Work out the finished part from the listing and answer in its coordinate system (mm). Face numbers are marked on the shaded views. A direction names the side the tool comes from. Coordinates: 2 decimals unless noted, no trailing zeros. Order: outer loops, then holes, each group sorted by start corner. A loop starts at its lowest first (then second) coordinate and runs counter-clockwise, first axis right, second up. Notation, with made-up numbers: (49, 60.5) -> (66, 60.5) arc R24 cw to (66, 91.5) -> close; hole circle Ø4 at (55, 6). An arc over 180 degrees is marked (long way). Answer as CSV lines item,"result". Start each with the question number.
Item 1: Section B-B (y = -30) is taken. Write down the section's boundary in (x, z), then the cut area to 3 significant figures.
Item 2: Which of the six approach directions +Z, -Z, +X, -X, +Y, -Y give full straight-line access (tool end or side, diameter ignored) to the marked faces 1 and 2?
Item 3: Section D-D (y = -9) is taken. Write down the section's boundary in (x, z).
Item 4: For a pull along Z with two mould halves and no side action, classify the marked faces 3, 4, 5 and 6 as pulls with the +Z half, pulls with the -Z half, needs draft (parallel to the pull), parting line crosses it, or undercut.
Item 5: Straight lines are drawn through the part: L1, parallel to X at y = -28, z = 0; L2, parallel to Z at x = -22.5, y = -33; L3, parallel to X at y = -10, z = 19. For each, find the intervals that lie inside material, in ascending order.
Item 6: Section C-C (x = -26) is taken. Write down the section's boundary in (y, z).
Item 7: Each of these flat-tipped pins is pushed along its axis until it touches: pin 1 Ø12 at (x, z) = (-53.5, -6.5) entering from -Y; pin 2 Ø12 at (y, z) = (-39, 24) entering from -X; pin 3 Ø8 at (y, z) = (-53, 54) entering from -X. Where does it stop, or does it pass through?
Item 8: Section A-A (z = 0) is taken. Write down the section's boundary in (x, y), then the cut area to 3 significant figures.
```python
from build123d import *

# Parameters (mm, degrees)
F0_W     = 10
F0_H     = 30
F1_DEPTH = 60
F2_R     = 10.2
F3_DEPTH = 80
F4_SIZE2 = 5
F4_SIZE  = 1


with BuildPart() as f1:
    # F0 (on Front) → F1 (new body)
    with BuildSketch(Plane.XZ):
        Polygon((5.41889066, 74.0884651807), (-5, 15), (5, 15), (15.41889066, 74.0884651807), align=None)
        Rectangle(F0_W, F0_H)
        Polygon((5, -15), (-5, -15), (5.41889066, -74.0884651807), (15.41889066, -74.0884651807), align=None)
    extrude(amount=F1_DEPTH)

    # F2 (on face) → F3 (join)
    with BuildSketch(Plane(origin=(-5, 0, 0), x_dir=(0, -1, 0), z_dir=(-1, 0, 0))):
        with Locations((30, 0)):
            Circle(F2_R)
    extrude(amount=F3_DEPTH)

    # F4
    f4_edges = [f1.edges().sort_by_distance(p)[0] for p in [
        (-85, -19.8, 0),
    ]]
    f4_side = f1.faces().sort_by_distance((-85, -30, 0))[0]
    chamfer(f4_edges, length=F4_SIZE, length2=F4_SIZE2, reference=f4_side)


solid = f1.part
```
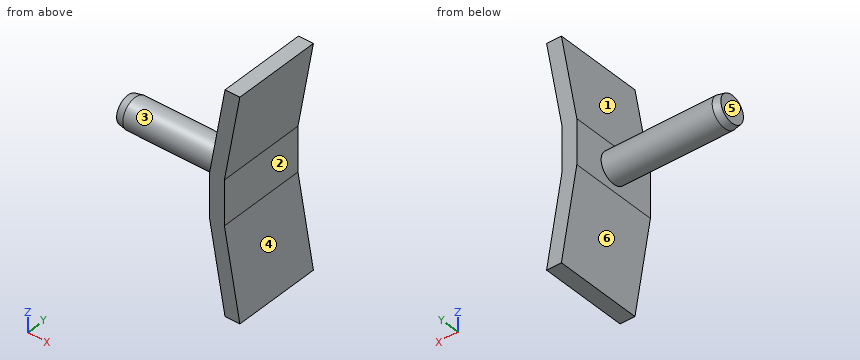
Checked values:
1,outline,"(-85, -9.2) -> (-80, -10.2) -> (-5, -10.2) -> (-5, -15) -> (5.42, -74.09) -> (15.42, -74.09) -> (5, -15) -> (5, 15) -> (15.42, 74.09) -> (5.42, 74.09) -> (-5, 15) -> (-5, 10.2) -> (-80, 10.2) -> (-85, 9.2) -> close"
1,area,"3,110 mm^2"
2,face 1,"+Z, -X, +Y, -Y"
2,face 2,"+X, +Y, -Y"
3,outline,"(-5, -15) -> (5.42, -74.09) -> (15.42, -74.09) -> (5, -15) -> (5, 15) -> (15.42, 74.09) -> (5.42, 74.09) -> (-5, 15) -> close"
4,face 3,"parting line crosses it"
4,face 4,"undercut"
4,face 5,"needs draft"
4,face 6,"pulls with the -Z half"
5,L1,"x = -85 to 5"
5,L2,"z = -9.75 to 9.75"
5,L3,"x = -4.29 to 5.71"
6,outline,"circle Ø20.4 at (-30, 0)"
7,pin 1,"stops at y = -40.19"
7,pin 2,"stops at x = -4.47"
7,pin 3,"stops at x = 1.17"
8,outline,"(-85, -39.2) -> (-80, -40.2) -> (-5, -40.2) -> (-5, -60) -> (5, -60) -> (5, 0) -> (-5, 0) -> (-5, -19.8) -> (-80, -19.8) -> (-85, -20.8) -> close"
8,area,"2,230 mm^2"
